Model file for the job. Use its own axes, mm. A direction names the side the tool comes from. Coordinates: 2 decimals unless noted, no trailing zeros. Loops run counter-clockwise (first coordinate to the right, second up) from the corner with the lowest first, then second, coordinate; pieces in that order, holes last. Notation, with made-up numbers: M 77,-24.5 L 109,-24.5 A15 cw 109,2.5 Z; hole C 13.5,47 d10. An arc over 180 degrees is marked long. One line per question, with ' | ' between items. Start each with the question number.
```python
from build123d import *

# Parameters (mm, degrees)
SKETCH1_R                  = 12.7
BOSS_EXTRUDE1_DEPTH        = 5.08
SKETCH2_R                  = 6.035
BOSS_EXTRUDE2_DEPTH        = 4.13
CUT_EXTRUDE1_REACH         = 22.184
SKETCH3_R                  = 3.1
SKETCH16_R                 = 2.05
CUT_EXTRUDE2_DEPTH         = 0.5
F_4_40_TAPPED_HOLE3_REACH  = 26.055
F_4_40_TAPPED_HOLE3_BORE_R = 1.1303
SKETCH24_R                 = 2.05
CUT_EXTRUDE3_DEPTH         = 7.1
F_4_40_TAPPED_HOLE4_REACH  = 26.104
F_4_40_TAPPED_HOLE4_BORE_R = 1.1303
SKETCH29_R                 = 1.5
CUT_EXTRUDE4_DEPTH         = 10


with BuildPart() as part:
    # Sketch1 → Boss-Extrude1 (new body)
    with BuildSketch(Plane.XY):
        Circle(SKETCH1_R)
    extrude(amount=BOSS_EXTRUDE1_DEPTH)

    # Sketch2 → Boss-Extrude2 (add)
    with BuildSketch(Plane.XY.offset(5.08)):
        Circle(SKETCH2_R)
    extrude(amount=BOSS_EXTRUDE2_DEPTH)

    # Sketch3 → Cut-Extrude1 (cut, up to next)
    with BuildSketch(Plane.XY.offset(9.21), mode=Mode.PRIVATE) as cut_extrude1_sk1:
        Circle(SKETCH3_R)
    cut_extrude1_tool1 = extrude(cut_extrude1_sk1.sketch, amount=-CUT_EXTRUDE1_REACH, mode=Mode.PRIVATE) & part.part
    add(cut_extrude1_tool1.solids().sort_by_distance((0, 0, 9.21))[0], mode=Mode.SUBTRACT)

    # Sketch16 → Cut-Extrude2 (cut)
    with BuildSketch(Plane(origin=(6.035, 0, 9.21), x_dir=(0, 0, -1), z_dir=(1, 0, 0))):
        with Locations(Location((2.069027283, 0, 0), (0, 0, 90))):
            Circle(SKETCH16_R)
    extrude(amount=-CUT_EXTRUDE2_DEPTH, mode=Mode.SUBTRACT)

    # #4-40 Tapped Hole3 bore → #4-40 Tapped Hole3 (cut, up to next)
    with BuildSketch(Plane(origin=(5.535, 0, 0), x_dir=(0, 0, -1), z_dir=(1, 0, 0)), mode=Mode.PRIVATE) as f_4_40_tapped_hole3_sk1:
        with Locations((-7.140972717, 0)):
            Circle(F_4_40_TAPPED_HOLE3_BORE_R)
    f_4_40_tapped_hole3_tool1 = extrude(f_4_40_tapped_hole3_sk1.sketch, amount=-F_4_40_TAPPED_HOLE3_REACH, mode=Mode.PRIVATE) & part.part
    add(f_4_40_tapped_hole3_tool1.solids().sort_by_distance((5.535, 0, 7.140973))[0], mode=Mode.SUBTRACT)

    # Sketch24 → Cut-Extrude3 (cut)
    with BuildSketch(Plane(origin=(12.7, 0, 5.08), x_dir=(0, 0, -1), z_dir=(1, 0, 0))):
        with Locations(Location((2.585319139, 0, 0), (0, 0, 90))):
            Circle(SKETCH24_R)
    extrude(amount=-CUT_EXTRUDE3_DEPTH, mode=Mode.SUBTRACT)

    # #4-40 Tapped Hole4 bore → #4-40 Tapped Hole4 (cut, up to next)
    with BuildSketch(Plane(origin=(5.6, 0, 0), x_dir=(0, 0, -1), z_dir=(1, 0, 0)), mode=Mode.PRIVATE) as f_4_40_tapped_hole4_sk1:
        with Locations((-2.494680861, 0)):
            Circle(F_4_40_TAPPED_HOLE4_BORE_R)
    f_4_40_tapped_hole4_tool1 = extrude(f_4_40_tapped_hole4_sk1.sketch, amount=-F_4_40_TAPPED_HOLE4_REACH, mode=Mode.PRIVATE) & part.part
    add(f_4_40_tapped_hole4_tool1.solids().sort_by_distance((5.6, 0, 2.494681))[0], mode=Mode.SUBTRACT)

    # Sketch29 → Cut-Extrude4 (cut)
    with BuildSketch(Plane.XY.offset(5.08)):
        with Locations((0, 9.5)):
            Circle(SKETCH29_R)
        with Locations((8.227241336, 4.75)):
            Circle(SKETCH29_R)
        with Locations((8.227241336, -4.75)):
            Circle(SKETCH29_R)
        with Locations((0, -9.5)):
            Circle(SKETCH29_R)
        with Locations((-8.227241336, -4.75)):
            Circle(SKETCH29_R)
        with Locations((-8.227241336, 4.75)):
            Circle(SKETCH29_R)
    extrude(amount=-CUT_EXTRUDE4_DEPTH, mode=Mode.SUBTRACT)


solid = part.part
```
(1) 3-axis set-ups, long thin cutter, end or side, ignore diameter. For faces 4 (the face through (-4.79, -3.67, 7.12)), 5 (the face through (4.23, 0.05, 8.27)), 6 (the face through (3, -3, 0)): which of +Z, -Z, +X, -X, +Y, -Y reach the whole face in a straight line?
(2) Two-plate mould, pull along X, no slides. Class faces 1 (the face through (5.6, 0, 1)), 2 (the face through (4.262, 0.05, 3.624)), 3 (the face through (-9.726, 4.816, 2.576)): pulls with the +X half, pulls with the -X half, needs draft (parallel to the pull), parting line crosses it, or undercut.
(3) Pin check, flat tips, straight feed: P1, Ø4, axis at x = 5, z = 2, coming from the +Y side; P2, Ø3, axis at x = -2.5, z = 2, coming from the -Y side; P3, Ø2.5, axis at y = 0, z = 7.14, coming from the +X side (3 decimals). Stop position of each tip, or through.
(4) Band-saw the part on A-A on y = 0. Write the cut outline in (x, z) (3 decimals).
(5) Band-saw the part on B-B on x = -8.25. Write the cut outline in (y, z), then the cut area to 3 significant figures.
(6) Band-saw the part on C-C on x = 0. Write the cut outline in (y, z) (3 decimals).
(7) Band-saw the part on D-D on y = -4.75. Write the cut outline in (x, z), then the cut area to 3 significant figures.
(8) Drill centre lines: line 1 (Z direction, x = 3.4, y = 0); line 2 (Z direction, x = 7, y = 0); line 3 (Y direction, x = -9, z = 0.5). Where is each one in solid material? Low to high. Write a range as [from, to].
Computed values:
1) face 4: +Z | face 5: +X | face 6: -Z, +X, -X, +Y, -Y
2) face 1: pulls with the +X half | face 2: needs draft | face 3: undercut
3) P1: y = 12.34 | P2: y = -12.66 | P3: x = 5.535
4) outline: M -12.7,0 L -3.1,0 L -3.1,9.21 L -6.035,9.21 L -6.035,5.08 L -12.7,5.08 Z; M 3.1,0 L 12.7,0 L 12.7,0.445 L 5.6,0.445 L 5.6,1.364 L 3.1,1.364 Z; M 3.1,3.625 L 5.6,3.625 L 5.6,4.545 L 12.7,4.545 L 12.7,5.08 L 6.035,5.08 L 6.035,5.091 L 5.535,5.091 L 5.535,6.011 L 3.1,6.011 Z; M 3.1,8.271 L 5.535,8.271 L 5.535,9.191 L 6.035,9.191 L 6.035,9.21 L 3.1,9.21 Z
5) outline: M -9.66,0 L -6.25,0 L -6.25,5.08 L -9.66,5.08 Z; M -3.25,0 L 3.25,0 L 3.25,5.08 L -3.25,5.08 Z; M 6.25,0 L 9.66,0 L 9.66,5.08 L 6.25,5.08 Z | area: 67.6 mm^2
6) outline: M -12.7,0 L -11,0 L -11,5.08 L -12.7,5.08 Z; M -8,0 L -3.1,0 L -3.1,9.21 L -6.035,9.21 L -6.035,5.08 L -8,5.08 Z; M 3.1,0 L 8,0 L 8,5.08 L 6.035,5.08 L 6.035,9.21 L 3.1,9.21 Z; M 11,0 L 12.7,0 L 12.7,5.08 L 11,5.08 Z
7) outline: M -11.78,0 L -9.73,0 L -9.73,5.08 L -11.78,5.08 Z; M -6.73,0 L 6.73,0 L 6.73,5.08 L 3.72,5.08 L 3.72,9.21 L -3.72,9.21 L -3.72,5.08 L -6.73,5.08 Z; M 9.73,0 L 11.78,0 L 11.78,5.08 L 9.73,5.08 Z | area: 120 mm^2
8) line 1: [0, 1.36], [3.62, 6.01], [8.27, 9.21] | line 2: [0, 0.44], [4.54, 5.08] | line 3: [-8.96, -6.04], [-3.46, 3.46], [6.04, 8.96]
